Source: three-view drawing plus pictorial views. Frame: mm from the lowest corner of the part. A direction names the side the tool comes from. Coordinates: 2 decimals unless noted, no trailing zeros. Order: outer loops, then holes, each group sorted by start corner. A loop starts at its lowest first (then second) coordinate and runs counter-clockwise, first axis right, second up. Notation, with made-up numbers: (-17.75, 24) - (17.25, 24) arc R31 ccw to (17.25, 62) - close; hole circle Ø9 at (33, -18.75). An arc over 180 degrees is marked (long way). Use a Markdown table: item, result. Add a question column.
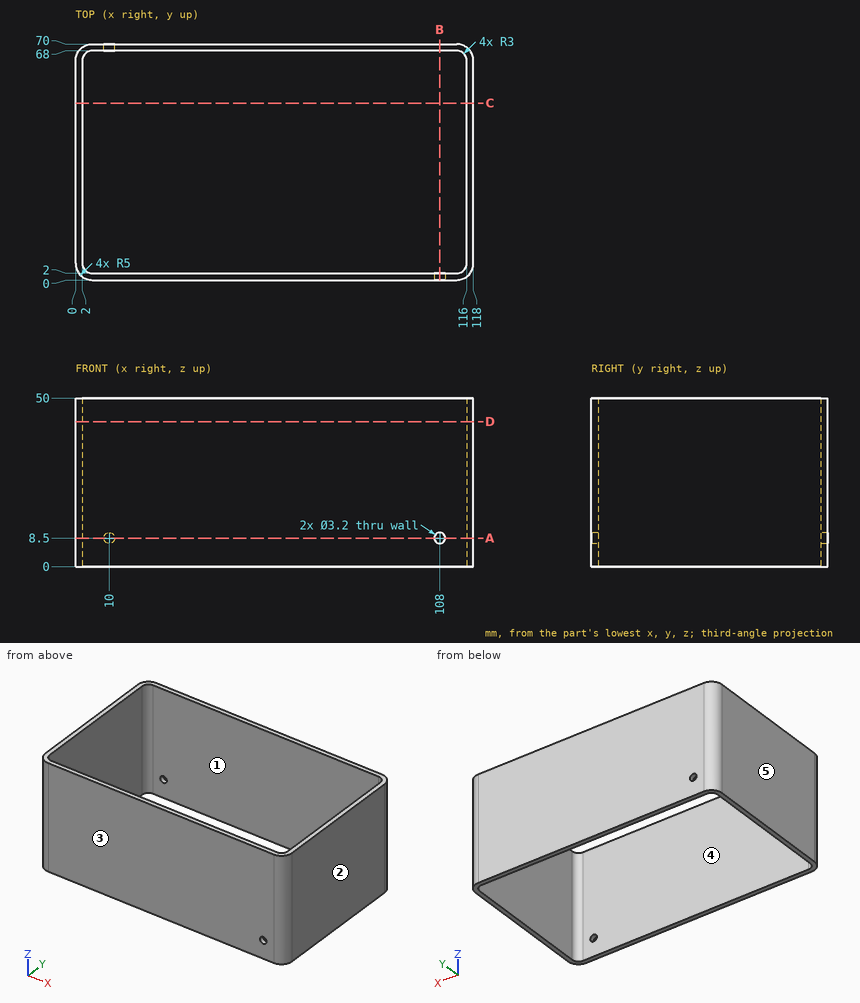
1) Pin query (flat end, axial travel): pin 1 (3 mm diameter, centred on x = 10, z = 8.5, fed in from +Y). Return the tip coordinate at first contact, or that it passes through.
2) Section C-C (y = 52.5). Return loops of the section in (x, z).
3) Section D-D (z = 43). Return loops of the section in (x, y), then the cut area to 3 significant figures.
4) Set-up query: the marked faces 4 and 5. Return all of +Z, -Z, +X, -X, +Y, -Y with unobstructed straight access to the full face (end or side cutting, diameter ignored); none if empty.
5) Draft query along Y for the marked faces 1, 2 and 3. Return one class per face: pulls with the +Y half, pulls with the -Y half, needs draft (parallel to the pull), parting line crosses it, or undercut.
6) Section B-B (x = 108). Return loops of the section in (y, z), then the cut area to 3 significant figures.
7) Section A-A (z = 8.5). Return loops of the section in (x, y), then the cut area to 3 significant figures.
8) Ray query, line 1 along Z through (x, y) = (108, 0.75); line 2 along X through (y, z) = (47.5, 45); line 3 along Y through (x, z) = (35, 31). Return the intervals inside material, ascending.
Values follow:
| question | item | result |
|---|---|---|
| 1 | pin 1 | stops at y = 2 |
| 2 | outline | (0, 0) - (2, 0) - (2, 50) - (0, 50) - close; (116, 0) - (118, 0) - (118, 50) - (116, 50) - close |
| 3 | outline | (0, 5) arc R5 ccw to (5, 0) - (113, 0) arc R5 ccw to (118, 5) - (118, 65) arc R5 ccw to (113, 70) - (5, 70) arc R5 ccw to (0, 65) - close; hole (2, 5) arc R3 ccw to (5, 2) - (113, 2) arc R3 ccw to (116, 5) - (116, 65) arc R3 ccw to (113, 68) - (5, 68) arc R3 ccw to (2, 65) - close |
| 3 | area | 722 mm² |
| 4 | face 4 | +Z, -Z |
| 4 | face 5 | +Z, -Z, -X, +Y, -Y |
| 5 | face 1 | undercut |
| 5 | face 2 | needs draft |
| 5 | face 3 | pulls with the -Y half |
| 6 | outline | (0, 0) - (2, 0) - (2, 6.9) - (0, 6.9) - close; (0, 10.1) - (2, 10.1) - (2, 50) - (0, 50) - close; (68, 0) - (70, 0) - (70, 50) - (68, 50) - close |
| 6 | area | 194 mm² |
| 7 | outline | (0, 5) arc R5 ccw to (5, 0) - (106.4, 0) - (106.4, 2) - (5, 2) arc R3 cw to (2, 5) - (2, 65) arc R3 cw to (5, 68) - (8.4, 68) - (8.4, 70) - (5, 70) arc R5 ccw to (0, 65) - close; (11.6, 68) - (113, 68) arc R3 cw to (116, 65) - (116, 5) arc R3 cw to (113, 2) - (109.6, 2) - (109.6, 0) - (113, 0) arc R5 ccw to (118, 5) - (118, 65) arc R5 ccw to (113, 70) - (11.6, 70) - close |
| 7 | area | 709 mm² |
| 8 | line 1 | z = 0 to 6.9, 10.1 to 50 |
| 8 | line 2 | x = 0 to 2, 116 to 118 |
| 8 | line 3 | y = 0 to 2, 68 to 70 |
